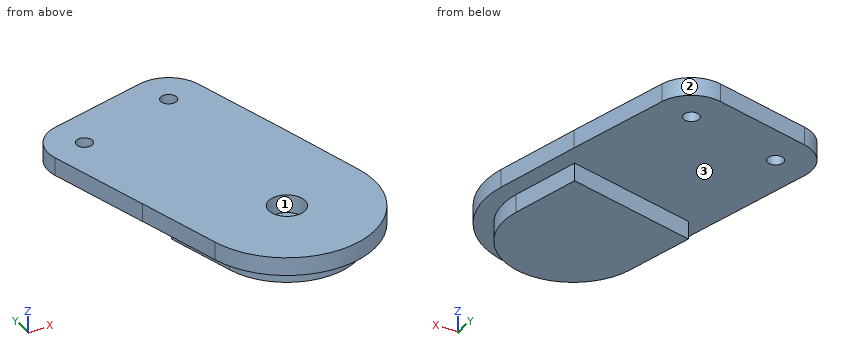
Autodesk Inventor part; units mm, degrees
ref_plane "YZ Plane" through (0, 0, 0) normal (1, 0, 0) x (0, 1, 0)
ref_plane "XZ Plane" through (0, 0, 0) normal (0, 1, 0) x (-1, 0, 0)
ref_plane "XY Plane" through (0, 0, 0) normal (0, 0, 1) x (1, 0, 0)
ref_plane "Work Plane1" through (0, 0, 0) normal (0, 0, 1) x (1, 0, 0)
sketch "Sketch1" plane through (0, 0, 0) normal (0, 0, 1) x (1, 0, 0)
  line L0 (-48.9636, -5.919) -> (-45.777, -18.2132)
  arc A0 (-45.777, -18.2132) -> (-22.1173, -12.3142) centre (-33.9472, -15.2637) ccw
  line L1 (-22.1173, -12.3142) -> (-25.2457, 0.2285)
  line L2 (-48.9636, -5.919) -> (-25.2457, 0.2285)
  point P0 (0, 0)
  point P1 (-37.0767, -2.9553)
  dimension "d0" = 12.2508
  dimension "d2" = 24.5017
  dimension "d3" = 12.7
extrude "Extrusion1" add sketch "Sketch1" along normal blind 3.175
sketch "Sketch2" plane through (0, 0, 3.175) normal (0, 0, 1) x (1, 0, 0)
  line L0 (-48.9636, -5.919) -> (-45.777, -18.2132)
  arc A0 (-45.777, -18.2132) -> (-22.1173, -12.3142) centre (-33.9472, -15.2637) ccw
  line L1 (-22.1173, -12.3142) -> (-25.2457, 0.2285)
  line L2 (-25.2457, 0.2285) -> (-48.9636, -5.919)
  line L3 (-48.9636, -5.919) -> (-45.777, -18.2132)
  arc A1 (-45.777, -18.2132) -> (-22.1173, -12.3142) centre (-33.9472, -15.2637) ccw
  line L4 (-22.1173, -12.3142) -> (-25.2457, 0.2285)
  line L5 (-25.2457, 0.2285) -> (-48.9636, -5.919)
  line L6 (-52.8328, -3.6427) -> (-48.8533, -18.9962)
  arc A2 (-48.8533, -18.9962) -> (-19.0376, -11.545) centre (-33.9472, -15.2637) ccw
  line L7 (-19.0376, -11.545) -> (-22.941, 4.1051)
  line L8 (-22.941, 4.1051) -> (-52.8328, -3.6427)
  line L9 (-52.8328, -3.72) -> (-22.941, 4.1051)
  line L10 (-22.941, 4.1051) -> (-29.388, 28.7327)
  line L11 (-29.388, 28.7327) -> (-59.2798, 20.9076)
  line L12 (-59.2798, 20.9076) -> (-52.8328, -3.72)
  point P0 (0, 0)
extrude "Extrusion2" add sketch "Sketch2" along normal blind 3.175 contours L2 L1 A0 L0 | L8 L9 L6 | L6 L9 L12 L11 L10 L8 | L9 L7 A2 L6
fillet "Fillet1" radius 6.35 2 edges at (-59.2798, 20.9076, 4.7625) (-29.388, 28.7327, 4.7625)
sketch "Sketch3" plane through (0, 0, 6.35) normal (0, 0, 1) x (1, 0, 0)
  circle A0 centre (-33.9229, -15.2576) radius 3.175
  point P0 (0, 0)
  dimension "d9" = 6.35
extrude "Extrusion3" cut sketch "Sketch3" against normal blind 3.175
sketch "Sketch4" plane through (0, 0, 6.35) normal (0, 0, 1) x (1, 0, 0)
  circle A0 centre (-51.5287, 16.3728) radius 1.397
  circle A1 centre (-33.9472, 20.9752) radius 1.397
  point P0 (0, 0)
  dimension "d12" = 2.794
  dimension "d13" = 2.794
extrude "Extrusion4" cut sketch "Sketch4" against normal up to next
properties part number "fingerBase01" material "Wood (Oak)"
Geometry: final body of the model. Coordinates: model frame, mm. Face numbers are marked on the shaded views. Give positions to 0.01 mm unless a question says otherwise; leave off trailing zeros. Loops run counter-clockwise (first coordinate to the right, second up) from the corner with the lowest first, then second, coordinate; pieces in that order, holes last. Notation, with made-up numbers: M -3,83 L 1,83 A32 cw 1,116 Z; hole C -16,34 d7. An arc over 180 degrees is marked long. Put each result on its own line as item: value.
1) Cut plane A-A, the plane y = -20. Return the cut outline in (x, z) (3 decimals).
Computed values:
outline: M -48.565,3.175 L -45.182,3.175 L -45.182,0 L -22.713,0 L -22.713,3.175 L -19.329,3.175 L -19.329,6.35 L -48.565,6.35 Z
2) Material intervals for L1, parallel to Z at x = -24.5, y = 9.5 (3 decimals); L2, parallel to X at y = 8.5, z = 4; L3, parallel to Y at x = -36, z = 4, sorted ascending. Write a range as from..to.
Computed values:
L1: z = 3.175..6.35
L2: x = -56.03..-24.09
L3: y = -30.49..-17.66, -12.86..27
3) First-contact query: P1, Ø1, axis at y = -12, z = 4, coming from the -X side; P2, Ø3, axis at x = -33, y = -15, coming from the +Z side (3 decimals); P3, Ø1.5, axis at y = -9.5, z = 4.5, coming from the -X side; P4, Ø5, axis at x = -33.92, y = -15.26, coming from the -Z side. Flat tips, straight axial feed; report the tip coordinate or a pass-through.
Computed values:
P1: stops at x = -50.8
P2: stops at z = 3.175
P3: stops at x = -51.51
P4: stops at z = 0
4) Cut plane B-B, the plane z = 4.25. Return the cut outline in (x, y) (3 decimals).
Computed values:
outline: M -57.672,14.765 L -52.833,-3.72 L -52.814,-3.715 L -48.853,-18.996 A15.366 ccw -19.038,-11.545 L -22.941,4.105 L -27.78,22.59 A6.35 ccw -35.531,27.125 L -53.137,22.516 A6.35 ccw Z; hole C -51.529,16.373 d2.794; hole C -33.923,-15.258 d6.35; hole C -33.947,20.975 d2.794
5) Cut plane C-C, the plane x = -47. Return the cut outline in (y, z) (3 decimals).
Computed values:
outline: M -23.372,3.175 L -13.495,3.175 L -13.495,0 L -5.41,0 L -5.41,3.175 L 24.122,3.175 L 24.122,6.35 L -23.372,6.35 Z
6) Cut plane D-D, the plane z = 1. Return the cut outline in (x, y).
Computed values:
outline: M -48.96,-5.92 L -45.78,-18.21 A12.19 ccw -22.12,-12.31 L -25.25,0.23 Z
7) Mould query, pull axis Y, two halves, no side actions, for the marked faces 1, 2 and 3. Classes: released by +Y, released by -Y, zero draft, split by the parting line, or undercut.
Computed values:
face 1: undercut
face 2: released by +Y
face 3: zero draft
